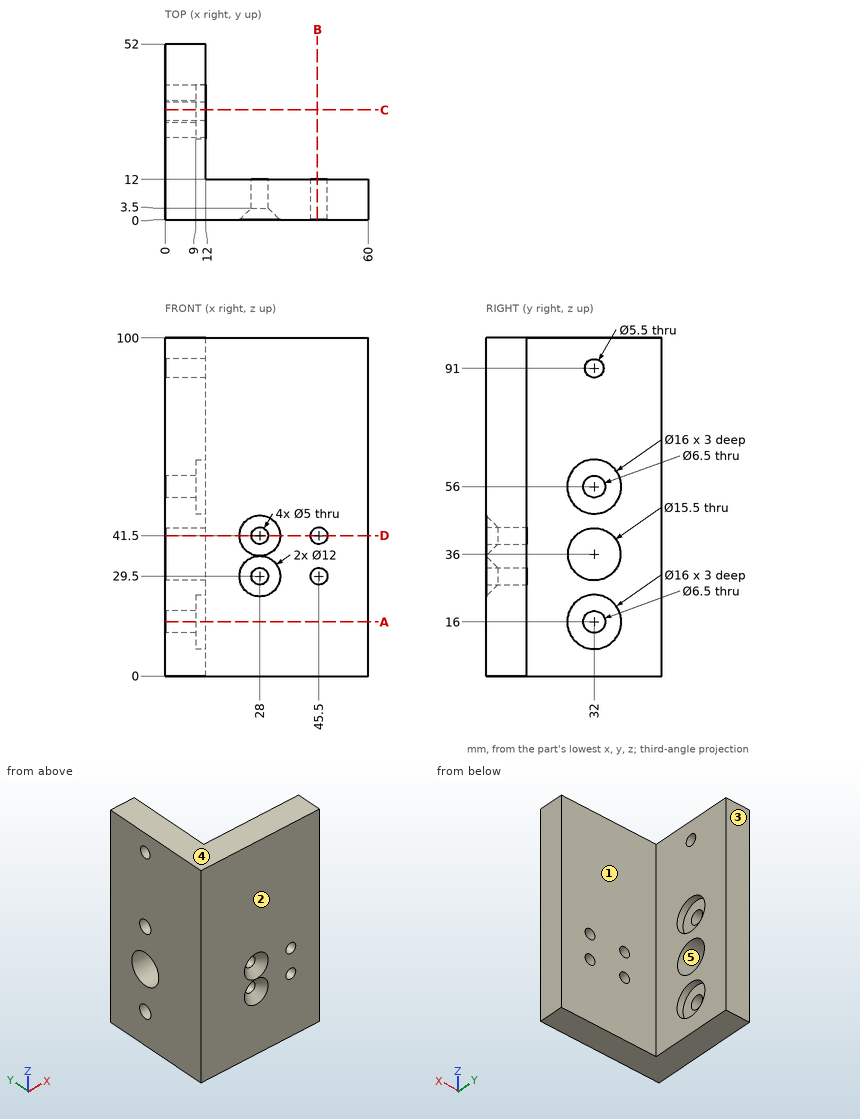
Study the drawing (mm; zero at the part's minimum x, y, z) and answer. A direction names the side the tool comes from. Give positions to 0.01 mm unless a question says otherwise; leave off trailing zeros. Write each loop counter-clockwise with the first axis right and the second up, starting at its lowest first coordinate (ties: lowest second). Pieces come first, ordered by that corner, then holes.
Item 1: Section D-D, the plane z = 41.5 is taken. Write down the section's boundary in (x, y).
Item 2: Flat-ended cylindrical pins translate along their axes: P1, Ø12, axis at y = 34.5, z = 65.5, coming from the +X side; P2, Ø10.5, axis at y = 32, z = 16, coming from the +X side; P3, Ø14.5, axis at x = 27, z = 39, coming from the +Y side. Find the tip coordinate at first contact, or state that the pin passes through.
Item 3: Which of the six approach directions +Z, -Z, +X, -X, +Y, -Y give full straight-line access (tool end or side, diameter ignored) to the marked faces 1 and 2?
Item 4: Section B-B, the plane x = 45 is taken. Write down the section's boundary in (y, z).
Item 5: Section A-A, the plane z = 16 is taken. Write down the section's boundary in (x, y).
Item 6: Determine the mould class of the marked faces 3, 4 and 5 for opening direction Z: released by +Z, released by -Z, zero draft, split by the parting line, or undercut.
Item 7: Section C-C, the plane y = 32.5 is taken. Write down the section's boundary in (x, z), plus the area to 3 significant figures.
Item 8: Find the intervals of material crossed by line 1 along Z through (x, y) = (7.25, 32); line 2 along Z through (x, y) = (28, 7.75); line 3 along Z through (x, y) = (10, 32), in increasing order.
Completed:
1. outline: (0, 0) - (22, 0) - (25.5, 3.5) - (25.5, 12) - (12, 12) - (12, 26.54) - (0, 26.54) - close; (0, 37.46) - (12, 37.46) - (12, 52) - (0, 52) - close; (30.5, 3.5) - (34, 0) - (43, 0) - (43, 12) - (30.5, 12) - close; (48, 0) - (60, 0) - (60, 12) - (48, 12) - close
2. P1: stops at x = 12
2. P2: stops at x = 9
2. P3: stops at y = 12
3. face 1: +Z, -Z, +X, +Y
3. face 2: +Z, -Z, +X, -X, -Y
4. outline: (0, 0) - (12, 0) - (12, 27.05) - (0, 27.05) - close; (0, 31.95) - (12, 31.95) - (12, 39.05) - (0, 39.05) - close; (0, 43.95) - (12, 43.95) - (12, 100) - (0, 100) - close
5. outline: (0, 0) - (60, 0) - (60, 12) - (12, 12) - (12, 24) - (9, 24) - (9, 28.75) - (0, 28.75) - close; (0, 35.25) - (9, 35.25) - (9, 40) - (12, 40) - (12, 52) - (0, 52) - close
6. face 3: zero draft
6. face 4: released by +Z
6. face 5: undercut
7. outline: (0, 0) - (12, 0) - (12, 8.02) - (9, 8.02) - (9, 12.79) - (0, 12.79) - close; (0, 19.21) - (9, 19.21) - (9, 23.98) - (12, 23.98) - (12, 28.27) - (0, 28.27) - close; (0, 43.73) - (12, 43.73) - (12, 48.02) - (9, 48.02) - (9, 52.79) - (0, 52.79) - close; (0, 59.21) - (9, 59.21) - (9, 63.98) - (12, 63.98) - (12, 88.3) - (0, 88.3) - close; (0, 93.7) - (12, 93.7) - (12, 100) - (0, 100) - close
7. area: 738 mm2
8. line 1: z = 0 to 12.75, 19.25 to 28.25, 43.75 to 52.75, 59.25 to 88.25, 93.75 to 100
8. line 2: z = 0 to 27, 32 to 39, 44 to 100
8. line 3: z = 0 to 8, 24 to 28.25, 43.75 to 48, 64 to 88.25, 93.75 to 100
